Geometry check sheet. Reference: drawing and pictorial views, mm from the part's lowest x, y, z. Round coordinates to 2 decimals unless told otherwise and drop trailing zeros. Write each loop counter-clockwise with the first axis right and the second up, starting at its lowest first coordinate (ties: lowest second). Pieces come first, ordered by that corner, then holes. Notation, with made-up numbers: M 27.25,82.5 L 70.25,82.5 A25 ccw 70.25,97.5 Z; hole C 49.25,78 d5. An arc over 180 degrees is marked long. One line per question, with ' | ' between items.
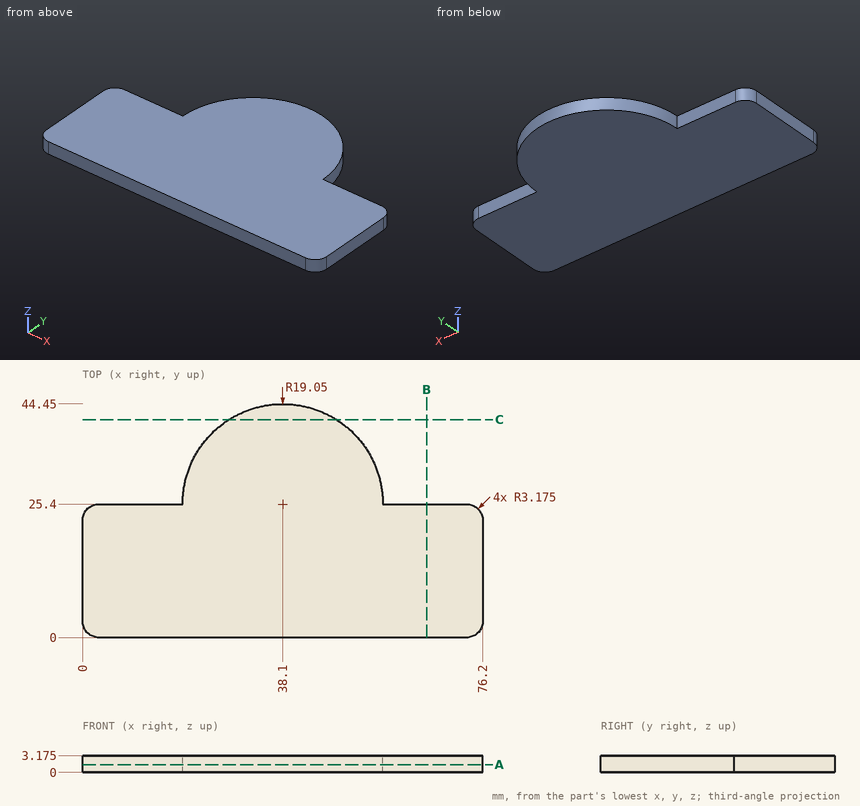
1. Thickness scan on line 1 (Y direction, x = 12, z = 2.45); line 2 (X direction, y = 3, z = 1.25); line 3 (Y direction, x = 40, z = 0.35). Record the ranges inside material, lowest first.
Results:
line 1: y = 0 to 25.4 | line 2: x = 0 to 76.2 | line 3: y = 0 to 44.36
2. Go/stop test with flat-tipped pins: P1, Ø1.5, axis at x = 31.5, z = 2.5, coming from the +Y side; P2, Ø1, axis at x = 8.5, z = 2, coming from the +Y side. Record where each tip stops, or that it passes through.
Results:
P1: stops at y = 43.53 | P2: stops at y = 25.4
3. Section check A-A, the plane z = 1.45. Record the cut outline in (x, y) (3 decimals).
Results:
outline: M 0,3.175 A3.175 ccw 3.175,0 L 73.025,0 A3.175 ccw 76.2,3.175 L 76.2,22.225 A3.175 ccw 73.025,25.4 L 57.15,25.4 A19.05 ccw 19.05,25.4 L 3.175,25.4 A3.175 ccw 0,22.225 Z
4. Section check C-C, the plane y = 41.5. Record the cut outline in (x, z) (3 decimals).
Results:
outline: M 27.917,0 L 48.283,0 L 48.283,3.175 L 27.917,3.175 Z
5. Section check B-B, the plane x = 65.5. Record the cut outline in (y, z) (3 decimals), then the cut area to 3 significant figures.
Results:
outline: M 0,0 L 25.4,0 L 25.4,3.175 L 0,3.175 Z | area: 80.6 mm2
